```python
from build123d import *

# Parameters (mm, degrees)
F0_W     = 381
F0_H     = 180.975
F1_DEPTH = 76.2
F2_W     = 317.5
F2_H     = 88.9
F3_DEPTH = 76.2
F4_SIZE  = 9.525
F5_SIZE  = 9.525


with BuildPart() as f1:
    # F0 (on Top) → F1 (new body)
    with BuildSketch(Plane.XY):
        with Locations((-2.829934, 34.121945)):
            Rectangle(F0_W, F0_H)
    extrude(amount=F1_DEPTH)

    # F2 (on face) → F3 (cut)
    with BuildSketch(Plane.XY.offset(76.2)):
        with Locations((-1.251158, 44.45)):
            Rectangle(F2_W, F2_H)
    extrude(amount=-F3_DEPTH, mode=Mode.SUBTRACT)

    # F4
    f4_edges = [f1.edges().sort_by_distance(p)[0] for p in [
        (-160.001158, 88.9, 38.1),
    ]]
    chamfer(f4_edges, length=F4_SIZE)

    # F5
    f5_edges = [f1.edges().sort_by_distance(p)[0] for p in [
        (157.498842, 0, 38.1),
    ]]
    chamfer(f5_edges, length=F5_SIZE)


solid = f1.part
```
Can you work these out from the model? Positions are in its coordinate system, mm. A direction names the side the tool comes from. Coordinates: 2 decimals unless noted, no trailing zeros. Loops run counter-clockwise (first coordinate to the right, second up) from the corner with the lowest first, then second, coordinate; pieces in that order, holes last. Notation, with made-up numbers: M -26,-25.75 L 33,-25.75 A35 cw 33,9.25 Z; hole C 53.5,-32 d4. An arc over 180 degrees is marked long. Put each result on its own line as item: value. Start each with the question number.
(1) I need wall thicknesses on probe 1 along X at (y, z) = (17, 47); probe 2 along Y at (x, z) = (-21.5, 13); probe 3 along X at (y, z) = (87, 49.5). Which ranges of each line are inside material? Lowest first, please.
(2) We'd pull the mould along Y, two halves only. Please class faces 3 (the face through (-5, -5, 76.2)), 4 (the face through (-5, 124.609, 38)), 5 (the face through (157.499, 49, 39)): +Y half, -Y half, draft (parallel to the pull), parting line (faces both ways), or undercut.
(3) Which directions (+Z, -Z, +X, -X, +Y, -Y) give clear straight access to the entire face, cutting with the end or side of a thin tool? Please do faces 1 (the face through (187.67, 33, 38)), 2 (the face through (-155.305, 84.071, 38.633)).
(4) Imagine slicing it at A-A on y = 27. List the corners of the cut face in (x, z) for me.
(5) Imagine slicing it at C-C on x = -39. List the corners of the cut face in (y, z) for me.
(6) Imagine slicing it at B-B on z = 24. List the corners of the cut face in (x, y) for me (3 decimals), and give its area (3 significant figures).
Worked answers:
1. probe 1: x = -193.33 to -160, 157.5 to 187.67
1. probe 2: y = -56.37 to 0, 88.9 to 124.61
1. probe 3: x = -193.33 to -152.38, 157.5 to 187.67
2. face 3: draft
2. face 4: +Y half
2. face 5: undercut
3. face 1: +Z, -Z, +X, +Y, -Y
3. face 2: +Z, -Z
4. outline: M -193.33,0 L -160,0 L -160,76.2 L -193.33,76.2 Z; M 157.5,0 L 187.67,0 L 187.67,76.2 L 157.5,76.2 Z
5. outline: M -56.37,0 L 0,0 L 0,76.2 L -56.37,76.2 Z; M 88.9,0 L 124.61,0 L 124.61,76.2 L 88.9,76.2 Z
6. outline: M -193.33,-56.366 L 187.67,-56.366 L 187.67,124.609 L -193.33,124.609 Z; hole M -160.001,0 L 147.974,0 L 157.499,9.525 L 157.499,88.9 L -150.476,88.9 L -160.001,79.375 Z
6. area: 40,800 mm2
